Can you work these out from the model? Positions are in its coordinate system, mm. A direction names the side the tool comes from. Give positions to 0.01 mm unless a question says otherwise; leave off trailing zeros. Loops run counter-clockwise (first coordinate to the right, second up) from the corner with the lowest first, then second, coordinate; pieces in that order, holes last. Notation, with made-up numbers: (-38, -9) - (-30, -9) arc R7 ccw to (-30, 3) - close; hole circle Ø6 at (18, 52.25). An arc over 180 degrees is marked (long way). Answer as a JSON object with one key per item and string values. Group by question number.
Item 1: Suppose I cut it at D-D on z = 0.75. Count the separate pieces of the cut face and the enclosed holes in it, and give its area (3 significant figures).
Item 2: Will these pins go through, and if not, where does the flat tip stop? pin 1 (12 mm diameter, centred on x = 6.5, y = 7.5, fed in from -Z); pin 2 (2 mm diameter, centred on y = 4, z = 0.5, fed in from +X); pin 3 (4.5 mm diameter, centred on x = -5, y = -8.66, fed in from -Z); pin 4 (3 mm diameter, centred on x = -6.5, z = -0.5, fed in from +Y).
Item 3: Suppose I cut it at C-C on y = -7.5. Write out the boundary of the cut face in (x, z), and give its area (3 significant figures).
Item 4: Which directions (+Z, -Z, +X, -X, +Y, -Y) give clear straight access to the entire face, cutting with the end or side of a thin tool? Please do faces 1 (the cylindrical face through (-4.658, -18.853, 1.521)), 2 (the flat face through (-16.179, -10.496, -1.972)), 3 (the flat face through (-1, 19, -2)).
Item 5: Suppose I cut it at A-A on x = -11. Write out the boundary of the cut face in (y, z), and give its area (3 significant figures).
Item 6: Thinking about a two-plate mould opening in X: for faces 4 (the cylindrical face through (31, -9.76, 1.48)), 5 (the cylindrical face through (-0.07, -5.75, -1.97)), 6 (the flat face through (-26.366, -15.239, -2.028)), which applies, pulls with the +X half, pulls with the -X half, needs draft (parallel to the pull), parting line crosses it, or undercut?
Item 7: Suppose I cut it at B-B on z = -3.25. Write out the boundary of the cut face in (x, y).
Item 8: Please list where these lines run through material, in increasing order: L1, parallel to X at y = 17, z = 1.5; L2, parallel to Y at x = 22, z = 0.7; L3, parallel to Y at x = 11, z = 0.8.
Autodesk Fusion 360 part; units mm, degrees
sketch "Skizze1" plane through (0, 0, 0) normal (0, 0, 1) x (1, 0, 0)
  circle A0 centre (0, 0) radius 32.5
  dimension "d1" = 65
extrude "Extrusion1" add sketch "Skizze1" along normal blind 3
sketch "Skizze2" plane through (0, 0, 0) normal (0, 0, -1) x (1, 0, 0)
  circle A0 centre (0, 0) radius 32.5
  circle A1 centre (0, 0) radius 5.75
  dimension "d4" = 11.5
extrude "Extrusion2" add sketch "Skizze2" along normal blind 4 contours A1
hole "Bohrung1" at (0, 0, 3) direction (0, 0, -1) diameter 4 depth 99 tip angle 118 counterbore diameter 8 counterbore depth 5
sketch "Skizze3" plane through (0, 0, 3) normal (0, 0, 1) x (-1, 0, 0)
  circle A0 centre (0, 0) radius 4
  circle A1 centre (0, 0) radius 32.5
  circle A2 centre (-10, 0.0001) radius 2.5
  circle A3 centre (-22, 0) radius 2.5
  circle A4 centre (-20, 7.5) radius 2.5
  circle A5 centre (-20, -7.5) radius 2.5
  circle A6 centre (-5, -8.6602) radius 2.5
  circle A7 centre (-16.4952, -13.5705) radius 2.5
  circle A8 centre (-11, -19.0526) radius 2.5
  circle A9 centre (-3.5048, -21.0705) radius 2.5
  circle A10 centre (5, -8.6603) radius 2.5
  circle A11 centre (3.5048, -21.0705) radius 2.5
  circle A12 centre (11, -19.0526) radius 2.5
  circle A13 centre (16.4952, -13.5705) radius 2.5
  circle A14 centre (10, -0.0001) radius 2.5
  circle A15 centre (20, -7.5) radius 2.5
  circle A16 centre (22, 0) radius 2.5
  circle A17 centre (20, 7.5) radius 2.5
  circle A18 centre (5, 8.6602) radius 2.5
  circle A19 centre (16.4952, 13.5705) radius 2.5
  circle A20 centre (11, 19.0526) radius 2.5
  circle A21 centre (3.5048, 21.0705) radius 2.5
  circle A22 centre (-5, 8.6603) radius 2.5
  circle A23 centre (-3.5048, 21.0705) radius 2.5
  circle A24 centre (-11, 19.0526) radius 2.5
  circle A25 centre (-16.4952, 13.5705) radius 2.5
  dimension "d12" = 5
  dimension "d13" = 10
  dimension "d14" = 5
  dimension "d15" = 12
  dimension "d18" = 5
  dimension "d19" = 5
  dimension "d21" = 360
extrude "Extrusion3" cut sketch "Skizze3" against normal blind 26 contours A2 | A3 | A4 | A5 | A6 | A7 | A8 | A9 | A10 | A11 | A12 | A13 | A14 | A15 | A16 | A17 | A18 | A19 | A20 | A21 | A22 | A23 | A24 | A25
sketch "Skizze4" plane through (0, 0, 0) normal (0, 0, -1) x (1, 0, 0)
  circle A0 centre (3.5048, -21.0705) radius 2.5
  circle A1 centre (22, 0) radius 2.5
  circle A2 centre (11, 19.0526) radius 2.5
  circle A3 centre (-5, -8.6603) radius 2.5
  circle A4 centre (-22, 0) radius 2.5
  circle A5 centre (-11, 19.0526) radius 2.5
  circle A6 centre (-5, 8.6602) radius 2.5
  circle A7 centre (-10, -0.0001) radius 2.5
  circle A8 centre (5, -8.6602) radius 2.5
  circle A9 centre (16.4952, 13.5705) radius 2.5
  circle A10 centre (20, -7.5) radius 2.5
  circle A11 centre (-3.5048, -21.0705) radius 2.5
  circle A12 centre (11, -19.0526) radius 2.5
  circle A13 centre (20, 7.5) radius 2.5
  circle A14 centre (10, 0.0001) radius 2.5
  circle A15 centre (-11, -19.0526) radius 2.5
  circle A16 centre (-20, 7.5) radius 2.5
  circle A17 centre (-3.5048, 21.0705) radius 2.5
  circle A18 centre (-16.4952, 13.5705) radius 2.5
  circle A19 centre (-16.4952, -13.5705) radius 2.5
  circle A20 centre (-20, -7.5) radius 2.5
  circle A21 centre (3.5048, 21.0705) radius 2.5
  circle A22 centre (16.4952, -13.5705) radius 2.5
  circle A23 centre (5, 8.6603) radius 2.5
  circle A24 centre (0, 0) radius 5.75
  circle A25 centre (0, 0) radius 32.5
  line L0 (1, -32.4807) -> (-1, -32.4807)
  line L1 (-1, -32.4807) -> (-1, -5)
  line L2 (-1, -5) -> (1, -5)
  line L3 (1, -5) -> (1, -32.4807)
  line L4 (28.6291, 15.3743) -> (4.8301, 1.634)
  line L5 (3.8301, 3.366) -> (27.6291, 17.1064)
  line L6 (27.6291, 17.1064) -> (28.6291, 15.3743)
  line L7 (4.8301, 1.634) -> (3.8301, 3.366)
  line L8 (-27.6291, 17.1064) -> (-3.8301, 3.366)
  line L9 (-4.8301, 1.634) -> (-28.6291, 15.3743)
  line L10 (-28.6291, 15.3743) -> (-27.6291, 17.1064)
  line L11 (-3.8301, 3.366) -> (-4.8301, 1.634)
  dimension "d25" = 360
extrude "Extrusion4" add sketch "Skizze4" along normal blind 4 contours A24 L4 L5 L6 | A24 L0 L1 L3 | A24 L8 L9 L10
chamfer "Fase1" distance 4 angle 45 3 edges at (0, 32.4807, -4) (28.1291, -16.2404, -4) (-28.1291, -16.2404, -4)
sketch "Skizze5" plane through (0, 0, 0) normal (0, 0, -1) x (1, 0, 0)
  circle A0 centre (3.5048, -21.0705) radius 2.5
  circle A1 centre (22, 0) radius 2.5
  circle A2 centre (11, 19.0526) radius 2.5
  circle A3 centre (-5, -8.6603) radius 2.5
  circle A4 centre (-22, 0) radius 2.5
  circle A5 centre (-11, 19.0526) radius 2.5
  circle A6 centre (-5, 8.6602) radius 2.5
  circle A7 centre (-10, -0.0001) radius 2.5
  circle A8 centre (5, -8.6602) radius 2.5
  circle A9 centre (16.4952, 13.5705) radius 2.5
  circle A10 centre (20, -7.5) radius 2.5
  circle A11 centre (-3.5048, -21.0705) radius 2.5
  circle A12 centre (11, -19.0526) radius 2.5
  circle A13 centre (20, 7.5) radius 2.5
  circle A14 centre (10, 0.0001) radius 2.5
  circle A15 centre (-11, -19.0526) radius 2.5
  circle A16 centre (-20, 7.5) radius 2.5
  circle A17 centre (-3.5048, 21.0705) radius 2.5
  circle A18 centre (-16.4952, 13.5705) radius 2.5
  circle A19 centre (-16.4952, -13.5705) radius 2.5
  circle A20 centre (-20, -7.5) radius 2.5
  circle A21 centre (3.5048, 21.0705) radius 2.5
  circle A22 centre (16.4952, -13.5705) radius 2.5
  circle A23 centre (5, 8.6603) radius 2.5
  circle A24 centre (0, 0) radius 32.5
  line L0 (-5.4038, 1.9652) -> (-28.6291, 15.3743)
  line L1 (-28.6291, 15.3743) -> (-27.6291, 17.1064)
  line L2 (-27.6291, 17.1064) -> (-4.4038, 3.6972)
  arc A25 (4.4038, 3.6972) -> (-4.4038, 3.6972) centre (0, 0) ccw
  line L3 (4.4038, 3.6972) -> (27.6291, 17.1064)
  line L4 (27.6291, 17.1064) -> (28.6291, 15.3743)
  line L5 (28.6291, 15.3743) -> (5.4038, 1.9652)
  arc A26 (1, -5.6624) -> (5.4038, 1.9652) centre (0, 0) ccw
  line L6 (1, -5.6624) -> (1, -32.4807)
  line L7 (1, -32.4807) -> (-1, -32.4807)
  line L8 (-1, -32.4807) -> (-1, -5.6624)
  arc A27 (-5.4038, 1.9652) -> (-1, -5.6624) centre (0, 0) ccw
Worked out:
{
 "1": {"separate pieces": "1", "enclosed holes": "25", "area": "2,800 mm2"},
 "2": {"pin 1": "stops at z = -4", "pin 2": "stops at x = 32.36", "pin 3": "passes through", "pin 4": "stops at y = 32.1"},
 "3": {"outline": "(-31.62, 0) - (-22.5, 0) - (-22.5, 3) - (-31.62, 3) - close; (-17.5, 0) - (-14.99, 0) - (-14.99, -4) - (-10.99, -4) - (-10.99, 0) - (-7.21, 0) - (-7.21, 3) - (-17.5, 3) - close; (-2.79, 0) - (2.79, 0) - (2.79, 3) - (-2.79, 3) - close; (7.21, 0) - (10.99, 0) - (10.99, -4) - (14.99, -4) - (14.99, 0) - (17.5, 0) - (17.5, 3) - (7.21, 3) - close; (22.5, 0) - (31.62, 0) - (31.62, 3) - (22.5, 3) - close", "area": "165 mm2"},
 "4": {"face 1": "+Z, -Z", "face 2": "-Z, -Y", "face 3": "-Z, -X, +Y"},
 "5": {"outline": "(-30.58, 0) - (-21.55, 0) - (-21.55, 3) - (-30.58, 3) - close; (-16.55, 0) - (-7.51, 0) - (-7.51, -4) - (-5.2, -4) - (-5.2, 0) - (-2.29, 0) - (-2.29, 3) - (-16.55, 3) - close; (2.29, 0) - (16.55, 0) - (16.55, 3) - (2.29, 3) - close; (21.55, 0) - (30.58, 0) - (30.58, 3) - (21.55, 3) - close", "area": "149 mm2"},
 "6": {"face 4": "parting line crosses it", "face 5": "undercut", "face 6": "pulls with the -X half"},
 "7": {"outline": "(-25.82, -13.75) - (-24.82, -15.48) - (-4.4, -3.7) arc R5.75 ccw to (4.4, -3.7) - (24.82, -15.48) - (25.82, -13.75) - (5.4, -1.97) arc R5.75 ccw to (1, 5.66) - (1, 29.23) - (-1, 29.23) - (-1, 5.66) arc R5.75 ccw to (-5.4, -1.97) - close; hole circle Ø4 at (0, 0)"},
 "8": {"L1": "x = -27.7 to -12.43, -9.57 to 9.57, 12.43 to 27.7", "L2": "y = -23.92 to -9, -6 to -2.5, 2.5 to 6, 9 to 23.92", "L3": "y = -30.58 to -21.55, -16.55 to -2.29, 2.29 to 16.55, 21.55 to 30.58"}
}
